from build123d import *

# Parameters (mm, degrees)
F0_W     = 500
F0_H     = 300
F0_W_2   = 489.9999916553
F0_H_2   = 289.9999916553
F1_DEPTH = 5
F2_DEPTH = 350


with BuildPart() as f1:
    # F0 (on Top) → F1 (new body)
    with BuildSketch(Plane.XY):
        Rectangle(F0_W, F0_H)
        Rectangle(F0_W_2, F0_H_2, mode=Mode.SUBTRACT)
        Rectangle(F0_W_2, F0_H_2)
    extrude(amount=-F1_DEPTH)

    # F0 (on Top) → F2 (join)
    with BuildSketch(Plane.XY):
        Rectangle(F0_W, F0_H)
        Rectangle(F0_W_2, F0_H_2, mode=Mode.SUBTRACT)
    extrude(amount=F2_DEPTH)


solid = f1.part
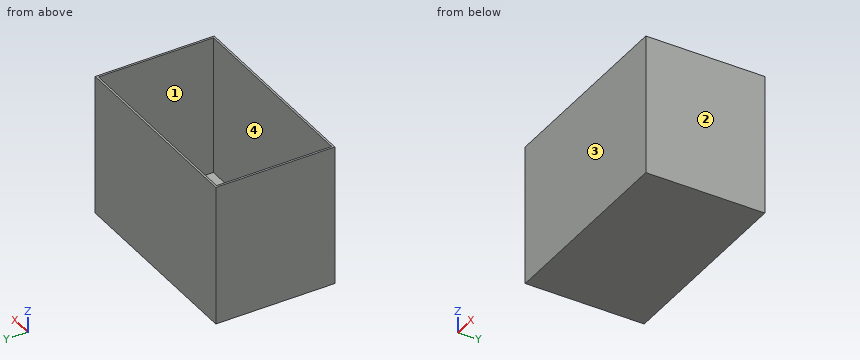
CAD build for the part. Positions are in the model's coordinates, mm. Face numbers are marked on the shaded views. Coordinates: 2 decimals unless noted, no trailing zeros. Write each loop counter-clockwise with the first axis right and the second up, starting at its lowest first coordinate (ties: lowest second). Pieces come first, ordered by that corner, then holes. Notation, with made-up numbers: M 65.5,43.25 L 92.5,43.25 A25 cw 92.5,59.25 Z; hole C -23,46 d7. An arc over 180 degrees is marked long. Return JSON: item names as keys, results as strings.
Item 1: Slice it at B-B, the plane y = 53. Write the cut outline in (x, z).
Findings below:
{"outline": "M -250,-5 L 250,-5 L 250,350 L 245,350 L 245,0 L -245,0 L -245,350 L -250,350 Z"}
Item 2: Probe line 1 (Y direction, x = -58, z = 24); line 2 (X direction, y = 99, z = 271); line 3 (Z direction, x = -187, y = -14.5). List the from-to ranges inside material, lowest first. Write a range as from..to.
Findings below:
{"line 1": "y = -150..-145, 145..150", "line 2": "x = -250..-245, 245..250", "line 3": "z = -5..0"}
Item 3: Slice it at A-A, the plane z = 91.5. Write the cut outline in (x, y).
Findings below:
{"outline": "M -250,-150 L 250,-150 L 250,150 L -250,150 Z; hole M -245,-145 L 245,-145 L 245,145 L -245,145 Z"}
Item 4: Drop a flat-ended pin along its axis: pin 1 Ø6 at (x, y) = (-141, -29.5) entering from +Z. Give the stop position or say it passes through.
Findings below:
{"pin 1": "stops at z = 0"}
Item 5: Slice it at C-C, the plane x = 192. Write the cut outline in (y, z), and give its area (3 significant figures).
Findings below:
{"outline": "M -150,-5 L 150,-5 L 150,350 L 145,350 L 145,0 L -145,0 L -145,350 L -150,350 Z", "area": "5,000 mm2"}
Item 6: Two-plate mould, pull along X, no slides. Class the marked faces 1, 2, 3 and 4: +X half, -X half, draft (parallel to the pull), parting line (faces both ways), or undercut.
Findings below:
{"face 1": "undercut", "face 2": "+X half", "face 3": "draft", "face 4": "undercut"}
